Work out the finished part from the listing and answer in its coordinate system (mm). A direction names the side the tool comes from. Coordinates: 2 decimals unless noted, no trailing zeros. Order: outer loops, then holes, each group sorted by start corner. A loop starts at its lowest first (then second) coordinate and runs counter-clockwise, first axis right, second up. Notation, with made-up numbers: M -17,14 L 34,14 A21 ccw 34,37 Z; hole C 31,-9.5 d10. An arc over 180 degrees is marked long. Use a Markdown table: item, result.
Autodesk Fusion 360 part; units mm, degrees
sketch "スケッチ1" plane through (0, 0, 0) normal (0, 0, 1) x (1, 0, 0)
  line L0 (-27.5, 6.35) -> (27.5, 6.35)
  line L1 (27.5, 6.35) -> (27.5, -6.35)
  line L2 (27.5, -6.35) -> (-27.5, -6.35)
  line L3 (-27.5, -6.35) -> (-27.5, 6.35)
  line L4 (-27.5, 6.35) -> (27.5, -6.35) construction
  line L5 (27.5, 6.35) -> (-27.5, -6.35) construction
  circle A0 centre (-12.5, -0.425) radius 1.75
  circle A1 centre (12.5, -0.425) radius 1.75
  dimension "d1" = 55
  dimension "d2" = 12.7
  dimension "d3" = 3.5
  dimension "d4" = 3.5
  dimension "d5" = 15
  dimension "d6" = 15
  dimension "d7" = 5.925
  dimension "d8" = 5.925
extrude "押し出し1" add sketch "スケッチ1" along normal blind 10 contours L0 L1 L2 L3 | A0 | A1
extrude "押し出し2" cut sketch "スケッチ1" along normal blind 6.6 contours A0 | A1
sketch "スケッチ2" plane through (0, 0, 10) normal (0, 0, 1) x (-1, 0, 0)
  line L0 (27.5, 6.35) -> (-27.5, 6.35)
  line L1 (-27.5, 6.35) -> (-27.5, -6.35)
  line L2 (-27.5, -6.35) -> (27.5, -6.35)
  line L3 (27.5, -6.35) -> (27.5, 6.35)
  circle A0 centre (12.5, 0.425) radius 3.25
  circle A1 centre (-12.5, 0.425) radius 3.25
  point P0 (12.5, 0.425)
  point P1 (-12.5, 0.425)
  dimension "d13" = 6.5
  dimension "d14" = 6.5
extrude "押し出し3" cut sketch "スケッチ2" against normal blind 3 contours A0 | A1
sketch "スケッチ3" plane through (0, 6.35, 0) normal (0, 1, 0) x (-1, 0, 0)
  line L0 (-27.5, 0) -> (27.5, 0)
  line L1 (27.5, 0) -> (27.5, 10)
  line L2 (27.5, 10) -> (-27.5, 10)
  line L3 (-27.5, 10) -> (-27.5, 0)
  circle A0 centre (0, -3.25) radius 8.1
  circle A1 centre (0, -3.25) radius 6.25
  line L4 (27.5, 0) -> (-27.5, 0)
  circle A2 centre (-21.5, -3.25) radius 5.5
  dimension "d17" = 16.2
  dimension "d18" = 12.5
  dimension "d19" = 3.25
  dimension "d20" = 11
  dimension "d21" = 3.25
  dimension "d22" = 6
extrude "押し出し4" cut sketch "スケッチ3" against normal through all contours L0 L4 A2 | L0 A1 L4 picked at (-21.5473, -2.9161) picked at (0.58, -6.8633)
extrude "押し出し5" cut sketch "スケッチ3" against normal blind 4 contours L0 A0 A1 L4 picked at (-6.9985, -0.6502)
extrude "押し出し6" cut sketch "スケッチ3" against normal up to surface (3.8 mm away) from surface at -8.9 contours L0 A0 A1 L4 picked at (-6.9985, -0.6502)
fillet "フィレット1" radius 1 4 edges at (-27.5, -6.35, 5) (-27.5, 6.35, 5) (27.5, -6.35, 5) (27.5, 6.35, 5)
equation "d8 = d7"
1. Find the intervals of material crossed by probe 1 along Y at (x, z) = (12.5, 8.95) (3 decimals); probe 2 along X at (y, z) = (1, 2.5); probe 3 along Y at (x, z) = (-12.5, 5.25) (3 decimals), in increasing order.
Answers below:
| item | result |
|---|---|
| probe 1 | -6.35 to -3.675, 2.825 to 6.35 |
| probe 2 | -27.5 to -13.52, -11.48 to 11.48, 13.52 to 27.5 |
| probe 3 | -6.35 to -2.175, 1.325 to 6.35 |
2. For a pull along X with two mould halves and no side action, classify faces 4 (the face through (27.199, -6.065, 5.07)), 5 (the face through (-27.199, 6.065, 5.07)), 6 (the face through (15.747, -0.568, 8.521)) as +X half, -X half, draft (parallel to the pull), parting line (faces both ways), or undercut.
Answers below:
| item | result |
|---|---|
| face 4 | +X half |
| face 5 | -X half |
| face 6 | undercut |
3. For faces 1 (the face through (-9.253, -0.568, 8.521)), 2 (the face through (27.215, 6.049, 5.07)), 3 (the face through (-13, 0, 6.6)), determine the directions among +Z, -Z, +X, -X, +Y, -Y from which every point of the face is accessible in a straight line to the end or side of a thin tool.
Answers below:
| item | result |
|---|---|
| face 1 | +Z |
| face 2 | +Z, -Z, +X, +Y |
| face 3 | -Z |
4. Section B-B on x = 12.5 is taken. Determine the outline of the cut face in (y, z) (3 decimals).
Answers below:
| item | result |
|---|---|
| outline | M -6.35,0 L -2.175,0 L -2.175,6.6 L 1.325,6.6 L 1.325,0 L 6.35,0 L 6.35,10 L 2.825,10 L 2.825,7 L -3.675,7 L -3.675,10 L -6.35,10 Z |
5. Section C-C on y = 0.25 is taken. Determine the outline of the cut face in (x, z), then the cut area to 3 significant figures.
Answers below:
| item | result |
|---|---|
| outline | M -27.5,0 L -14.11,0 L -14.11,6.6 L -10.89,6.6 L -10.89,0 L 10.89,0 L 10.89,6.6 L 14.11,6.6 L 14.11,0 L 27.5,0 L 27.5,10 L 15.68,10 L 15.68,7 L 9.32,7 L 9.32,10 L -9.32,10 L -9.32,7 L -15.68,7 L -15.68,10 L -27.5,10 Z |
| area | 469 mm² |
6. Flat-ended cylindrical pins translate along their axes: P1, Ø1.8, axis at x = 13, y = -0.5, coming from the -Z side; P2, Ø2, axis at x = 13.5, y = 0, coming from the +Z side. Find the tip coordinate at first contact, or state that the pin passes through.
Answers below:
| item | result |
|---|---|
| P1 | z = 6.6 |
| P2 | z = 7 |
7. Section A-A on z = 5.25 is taken. Determine the outline of the cut face in (x, y) (3 decimals).
Answers below:
| item | result |
|---|---|
| outline | M -27.5,-5.35 A1 ccw -26.5,-6.35 L 26.5,-6.35 A1 ccw 27.5,-5.35 L 27.5,5.35 A1 ccw 26.5,6.35 L -26.5,6.35 A1 ccw -27.5,5.35 Z; hole C -12.5,-0.425 d3.5; hole C 12.5,-0.425 d3.5 |
